Autodesk Inventor part; units mm, degrees
ref_plane "YZ Plane" through (0, 0, 0) normal (1, 0, 0) x (0, 1, 0)
ref_plane "XZ Plane" through (0, 0, 0) normal (0, 1, 0) x (-1, 0, 0)
ref_plane "XY Plane" through (0, 0, 0) normal (0, 0, 1) x (1, 0, 0)
sketch "Sketch1" plane through (0, 0, 0) normal (1, 0, 0) x (0, 1, 0)
  line L0 (0, 0) -> (76.2, 0)
  line L1 (76.2, 0) -> (76.2, -25.4)
  line L2 (76.2, -25.4) -> (0, -25.4)
  line L3 (0, -25.4) -> (0, 0)
  arc A0 (74.6125, -25.4) -> (42.8625, -25.4) centre (58.7375, -25.4) ccw
  dimension "d0" = 76.2
  dimension "d1" = 25.4
  dimension "d2" = 31.75
  dimension "d3" = 15.875
  dimension "d20" = 1.5875
extrude "Extrusion1" add sketch "Sketch1" along normal blind 6.35 contours L0 L1 L2 A0 L3
sketch "Sketch2" plane through (0, 0, -25.4) normal (0, -1, 0) x (1, 0, 0)
  line L0 (3.175, 21.59) -> (3.175, 3.81) construction
  line L1 (1.905, 20.32) -> (1.905, 5.08)
  line L2 (4.445, 5.08) -> (4.445, 20.32)
  arc A0 (4.445, 20.32) -> (1.905, 20.32) centre (3.175, 20.32) ccw
  arc A1 (1.905, 5.08) -> (4.445, 5.08) centre (3.175, 5.08) ccw
  line L3 (6.35, 25.4) -> (6.35, 0)
  line L4 (0, 25.4) -> (6.35, 25.4)
  point P0 (3.175, 12.7)
  dimension "d6" = 2.54
  dimension "d7" = 25.4
  dimension "d8" = 12.7
  dimension "d9" = 8.89
extrude "Extrusion2" cut sketch "Sketch2" against normal blind 38.1
sketch "Sketch4" plane through (6.35, 0, 0) normal (1, 0, 0) x (0, 0, -1)
  line L0 (5.08, 0) -> (5.08, 38.1)
  line L1 (0, 0) -> (25.4, 0)
  line L2 (25.4, 0) -> (25.4, 42.8625)
  arc A0 (25.4, 74.6125) -> (25.4, 42.8625) centre (25.4, 58.7375) ccw
  line L3 (25.4, 76.2) -> (0, 76.2)
  line L4 (0, 76.2) -> (0, 0)
  circle A1 centre (12.7, 39.7791) radius 0.635
  circle A2 centre (12.7, 39.7791) radius 3.048
  line L5 (25.4, 74.6125) -> (25.4, 76.2)
  dimension "d16" = 1.27
  dimension "d17" = 6.096
extrude "Extrusion4" add sketch "Sketch4" along normal blind 27.94 contours A2
properties part number "hook"
Verification items for the finished model (mm, model axes). A direction names the side the tool comes from. Coordinates: 2 decimals unless noted, no trailing zeros. Order: outer loops, then holes, each group sorted by start corner. A loop starts at its lowest first (then second) coordinate and runs counter-clockwise, first axis right, second up.
1. Sectioned sample at D-D, the plane x = 20. Record the cut outline in (y, z) (3 decimals), and give its area (3 significant figures).
Results found:
outline: circle Ø6.096 at (39.779, -12.7); hole circle Ø1.27 at (39.779, -12.7)
area: 27.9 mm2
2. Release check for a two-part mould opening along X. For faces 4 (the face through (4.445, 19, -13)), 5 (the face through (3, 38, 0)), 6 (the face through (6.35, 29, -10)), 7 (the face through (0, 29, -10)) record: +X half, -X half, draft (parallel to the pull), parting line (faces both ways), or undercut.
Results found:
face 4: undercut
face 5: draft
face 6: +X half
face 7: -X half
3. Sectioned sample at B-B, the plane z = -23.5. Record the cut outline in (x, y).
Results found:
outline: (0, 0) - (6.35, 0) - (6.35, 42.98) - (0, 42.98) - close; (0, 74.5) - (6.35, 74.5) - (6.35, 76.2) - (0, 76.2) - close
4. Set-up check for faces 1 (the face through (3, 38.1, -13)), 2 (the face through (3, 76.2, -13)), 3 (the face through (20.124, 42.755, -12.039)): record each of +Z, -Z, +X, -X, +Y, -Y from which the full face is reachable in a straight line by a thin tool's end or side.
Results found:
face 1: -Y
face 2: +Z, -Z, +X, -X, +Y
face 3: +X
5. Scan lines: line 1 (X direction, y = 6, z = -10.75) (3 decimals); line 2 (Y direction, x = 22.75, z = -12.7); line 3 (X direction, y = 72.5, z = -9.5). Record each from-to range of solid material in increasing order.
Results found:
line 1: x = 0 to 1.905, 4.445 to 6.35
line 2: y = 36.73 to 39.14, 40.41 to 42.83
line 3: x = 0 to 6.35
6. Go/stop test with flat-tipped pins: pin 1 Ø0.8 at (y, z) = (39.78, -12.7) entering from +X; pin 2 Ø1 at (y, z) = (39.5, -12.5) entering from +X; pin 3 Ø2 at (x, z) = (3, -16.5) entering from -Y; pin 4 Ø6 at (x, z) = (17, -11) entering from +Y. Record where each tip stops, or that it passes through.
Results found:
pin 1: stops at x = 6.35
pin 2: stops at x = 34.29
pin 3: stops at y = 38.1
pin 4: stops at y = 42.83
7. Sectioned sample at A-A, the plane y = 35.5. Record the cut outline in (x, z) (3 decimals).
Results found:
outline: (0, -25.4) - (6.35, -25.4) - (6.35, 0) - (0, 0) - close; hole (1.905, -20.32) arc R1.27 ccw to (4.445, -20.32) - (4.445, -5.08) arc R1.27 ccw to (1.905, -5.08) - close
